from build123d import *

# Parameters (mm, degrees)
F0_W     = 101.726
F0_H     = 97.916
F0_W_2   = 93.726
F0_H_2   = 89.916
F1_DEPTH = 13.97
F1_TAPER = 1
F2_T     = -4
F3_R     = 29.21
F3_R_2   = 25.4
F4_DEPTH = 12.7
F5_DEPTH = 4


with BuildPart() as f1:
    # F0 (on Front) → F1 (new body)
    with BuildSketch(Plane.XZ):
        Rectangle(F0_W, F0_H)
        Rectangle(F0_W_2, F0_H_2, mode=Mode.SUBTRACT)
        Rectangle(F0_W_2, F0_H_2)
    extrude(amount=F1_DEPTH, taper=F1_TAPER)

    # F2
    f2_openings = [f1.faces().sort_by_distance(p)[0] for p in [
        (0, -13.97, 0),
    ]]
    offset(amount=F2_T, openings=f2_openings)

    # F3 (on face) → F4 (join)
    with BuildSketch(Plane(origin=(0, 0, 0), x_dir=(-1, 0, 0), z_dir=(0, 1, 0))):
        Circle(F3_R)
        Circle(F3_R_2, mode=Mode.SUBTRACT)
    extrude(amount=F4_DEPTH)

    # F5 (cut, through all): a face of the model
    f5_faces = [f1.faces().sort_by_distance(p)[0] for p in [
        (0, 0, 0),
    ]]
    extrude(f5_faces, amount=-F5_DEPTH, mode=Mode.SUBTRACT)


solid = f1.part
Read the model definition and answer for the solid it produces. Units are mm, in the model's axes. A direction names the side the tool comes from. Round coordinates to 2 decimals unless told otherwise and drop trailing zeros. Write each loop counter-clockwise with the first axis right and the second up, starting at its lowest first coordinate (ties: lowest second). Pieces come first, ordered by that corner, then holes. Notation, with made-up numbers: (11, 35) - (41, 35) arc R12 ccw to (41, 42) - close; hole circle Ø2 at (1, 49.5). An arc over 180 degrees is marked (long way). Use a Markdown table: item, result.
(1) Each of these flat-tipped pins is pushed along its axis until it touches: pin 1 Ø10 at (x, z) = (-32, 24.5) entering from +Y; pin 2 Ø12 at (y, z) = (-6.5, 27) entering from -X; pin 3 Ø3 at (x, z) = (32, 36.5) entering from -Y. Where does it stop, or does it pass through?
Reported:
| item | result |
|---|---|
| pin 1 | y = 0 |
| pin 2 | x = -50.85 |
| pin 3 | y = -4 |
(2) Straight lines are drawn through the part: line 1 along Z through (x, y) = (0, 5); line 2 along Y through (x, z) = (28.5, 15); line 3 along Z through (x, y) = (-19.5, 3). For each, find the intervals that lie inside material, in ascending order. Write a range as [from, to].
Reported:
| item | result |
|---|---|
| line 1 | [-29.21, -25.4], [25.4, 29.21] |
| line 2 | [-4, 0] |
| line 3 | [-21.75, -16.28], [16.28, 21.75] |
(3) Which of the six approach directions +Z, -Z, +X, -X, +Y, -Y give full straight-line access (tool end or side, diameter ignored) to faces 5 (the flat face through (-23, 0, 23)), 6 (the flat face through (9, 12.7, 24))?
Reported:
| item | result |
|---|---|
| face 5 | +Y |
| face 6 | +Z, -Z, +X, -X, +Y |
(4) The part is cut by section A-A (y = 10.75). Write down the section's boundary in (x, z).
Reported:
| item | result |
|---|---|
| outline | circle Ø58.42 at (0, 0); hole circle Ø50.8 at (0, 0) |
(5) The mould has two halves that part along X. Classify faces 1 (the cylindrical face through (5.506, 4.233, -24.796)), 2 (the flat face through (19, -4, -21)), 3 (the flat face through (47, -13.97, -5)), 4 (the cylindrical face through (21.53, 6.26, 19.74)): released by +X, released by -X, zero draft, split by the parting line, or undercut.
Reported:
| item | result |
|---|---|
| face 1 | undercut |
| face 2 | undercut |
| face 3 | zero draft |
| face 4 | split by the parting line |
